Check sheet for the modelled part. Datum: model origin and axes. Units: mm. A direction names the side the tool comes from. Round coordinates to 2 decimals unless told otherwise and drop trailing zeros. Loops run counter-clockwise (first coordinate to the right, second up) from the corner with the lowest first, then second, coordinate; pieces in that order, holes last. Notation, with made-up numbers: (-17.75, 32) - (-9.75, 32) arc R18 cw to (-9.75, 46) - close; hole circle Ø5 at (86, -1). An arc over 180 degrees is marked (long way). Put each result on its own line as item: value. Start each with the question number.
```python
from build123d import *

# Parameters (mm, degrees)
F0_R     = 35.56
F1_DEPTH = 6.35
F2_R     = 35.56
F2_R_2   = 25.4
F3_DEPTH = 1.27
F4_SIZE  = 1.27
F5_R     = 21.59
F6_DEPTH = 25.4
F8_DEPTH = 6.35


with BuildPart() as f1:
    # F0 (on Top) → F1 (new body)
    with BuildSketch(Plane.XY):
        Circle(F0_R)
    extrude(amount=F1_DEPTH)

    # F2 (on face) → F3 (join)
    with BuildSketch(Plane.XY.offset(6.35)):
        Circle(F2_R)
        Circle(F2_R_2, mode=Mode.SUBTRACT)
    extrude(amount=F3_DEPTH)

    # F4
    f4_edges = [f1.edges().sort_by_distance(p)[0] for p in [
        (-35.56, 0, 0),
    ]]
    chamfer(f4_edges, length=F4_SIZE)

    # F5 (on face) → F6 (cut)
    with BuildSketch(Plane.XY.offset(6.35)):
        Circle(F5_R)
    extrude(amount=-F6_DEPTH, mode=Mode.SUBTRACT)

    # F7 (on face) → F8 (cut)
    with BuildSketch(Plane.XY.offset(7.62)):
        with BuildLine():
            ThreePointArc((-35.1952724098, 5.08), (-35.56, 0), (-35.1952724098, -5.08))
            Line((-35.1952724098, -5.08), (-24.8868157867, -5.08))
            ThreePointArc((-24.8868157867, -5.08), (-25.4, 0), (-24.8868157867, 5.08))
            Line((-24.8868157867, 5.08), (-35.1952724098, 5.08))
        make_face()
        with BuildLine():
            Line((-24.8868157867, -5.08), (24.8868157867, -5.08))
            ThreePointArc((24.8868157867, -5.08), (25.2713782863, -2.5529276349), (25.4, 0))
            ThreePointArc((25.4, 0), (25.2713782863, 2.5529276349), (24.8868157867, 5.08))
            Line((24.8868157867, 5.08), (-24.8868157867, 5.08))
            ThreePointArc((-24.8868157867, 5.08), (-25.4, 0), (-24.8868157867, -5.08))
        make_face()
        with BuildLine():
            Line((24.8868157867, -5.08), (35.1952724098, -5.08))
            ThreePointArc((35.1952724098, -5.08), (35.4687008988, -2.5465381509), (35.56, 0))
            ThreePointArc((35.56, 0), (35.4687008988, 2.5465381509), (35.1952724098, 5.08))
            Line((35.1952724098, 5.08), (24.8868157867, 5.08))
            ThreePointArc((24.8868157867, 5.08), (25.2713782863, 2.5529276349), (25.4, 0))
            ThreePointArc((25.4, 0), (25.2713782863, -2.5529276349), (24.8868157867, -5.08))
        make_face()
    extrude(amount=-F8_DEPTH, mode=Mode.SUBTRACT)


solid = f1.part
```
Q1. Depth check by flat-ended pin: pin 1 Ø5 at (x, y) = (12.5, 11.5) entering from -Z; pin 2 Ø2 at (x, z) = (11, 3) entering from +Y (3 decimals); pin 3 Ø1.9 at (x, z) = (-30, 5.5) entering from -Y; pin 4 Ø1.5 at (y, z) = (-25, 7) entering from +X. Enter the tip coordinate at first touch or a pass-through.
Q2. Cross-section at A-A on y = 0. Enter the section's corners in (x, z), and give its area (3 significant figures).
Q3. Set-up check for faces 4 (the face through (-28, 0, 1.27)), 5 (the face through (0, -27, 7.62)), 6 (the face through (0.487, 25.395, 6.976)): record each of +Z, -Z, +X, -X, +Y, -Y from which the full face is reachable in a straight line by a thin tool's end or side.
Q4. Cross-section at C-C on x = 0. Enter the section's corners in (y, z), and give its area (3 significant figures).
Q5. Material ranges on line 1 (Y direction, x = -3, z = 2.5); line 2 (X direction, y = 17, z = 1.25); line 3 (Y direction, x = -12, z = 4), recorded low to high. Write a range as from..to.
Q6. Cross-section at B-B on z = 5. Enter the section's corners in (x, y), and give its area (3 significant figures).
Q7. Draft check along Y on faces 1 (the face through (0, 27, 7.62)), 2 (the face through (28, -5.08, 4)), 3 (the face through (-0.711, -35.553, 4.401)). Enter one of: +Y half, -Y half, draft (parallel to the pull), parting line (faces both ways), or undercut.
Answer list:
1. pin 1: passes through
1. pin 2: stops at y = 34.125
1. pin 3: stops at y = -20.51
1. pin 4: stops at x = 26.01
2. outline: (-35.56, 1.27) - (-34.29, 0) - (-21.59, 0) - (-21.59, 1.27) - close; (21.59, 0) - (34.29, 0) - (35.56, 1.27) - (21.59, 1.27) - close
2. area: 33.9 mm2
3. face 4: +Z, +X, -X
3. face 5: +Z, +X, -X, +Y, -Y
3. face 6: +Z
4. outline: (-35.56, 1.27) - (-34.29, 0) - (-21.59, 0) - (-21.59, 6.35) - (-25.4, 6.35) - (-25.4, 7.62) - (-35.56, 7.62) - close; (21.59, 0) - (34.29, 0) - (35.56, 1.27) - (35.56, 7.62) - (25.4, 7.62) - (25.4, 6.35) - (21.59, 6.35) - close
4. area: 202 mm2
5. line 1: y = -35.43..-21.38, 21.38..35.43
5. line 2: x = -31.21..-13.31, 13.31..31.21
5. line 3: y = -33.47..-17.95, 17.95..33.47
6. outline: (-35.2, -5.08) arc R35.56 ccw to (35.2, -5.08) - (20.98, -5.08) arc R21.59 cw to (-20.98, -5.08) - close; (-35.2, 5.08) - (-20.98, 5.08) arc R21.59 cw to (20.98, 5.08) - (35.2, 5.08) arc R35.56 ccw to start
6. area: 2,220 mm2
7. face 1: draft
7. face 2: undercut
7. face 3: -Y half
